Input: part model. Units: mm. Frame: model coordinates. A direction names the side the tool comes from. Round coordinates to 2 decimals unless told otherwise and drop trailing zeros. Order: outer loops, then holes, each group sorted by start corner. A loop starts at its lowest first (then second) coordinate and runs counter-clockwise, first axis right, second up. Notation, with made-up numbers: M 28.5,25.25 L 62.5,25.25 A25 cw 62.5,41.25 Z; hole C -14.75,-20.75 d11. An arc over 180 degrees is marked long. One line per question, with ' | ' between items.
```python
from build123d import *

# Parameters (mm, degrees)
SKETCH1_W           = 30
SKETCH1_H           = 15
SKETCH1_R           = 1.5
SKETCH1_W_2         = 15
SKETCH1_H_2         = 17
SKETCH1_R_2         = 5
BOSS_EXTRUDE1_DEPTH = 5
SKETCH3_R           = 5
BOSS_EXTRUDE2_DEPTH = 15


with BuildPart() as part:
    # Sketch1 → Boss-Extrude1 (new body)
    # profile 1 of 3: a face of its own
    with BuildSketch(Plane(origin=(0, 0, 0), x_dir=(1, 0, 0), z_dir=(0, 1, 0))):
        with Locations((-15, -7.5)):
            Rectangle(SKETCH1_W, SKETCH1_H)
        with Locations(Location((-5, -7.5, 0), (0, 0, 270))):
            Circle(SKETCH1_R, mode=Mode.SUBTRACT)
        with Locations(Location((-25, -7.5, 0), (0, 0, 270))):
            Circle(SKETCH1_R, mode=Mode.SUBTRACT)
    # profile 2 of 3: a face of its own
    with BuildSketch(Plane(origin=(0, 0, 0), x_dir=(1, 0, 0), z_dir=(0, 1, 0))):
        with Locations((-15, 8.5)):
            Rectangle(SKETCH1_W_2, SKETCH1_H_2)
        with Locations((-15, 9)):
            Circle(SKETCH1_R_2, mode=Mode.SUBTRACT)
    # profile 3 of 3: a face of its own
    with BuildSketch(Plane(origin=(0, 0, 0), x_dir=(1, 0, 0), z_dir=(0, 1, 0))):
        with Locations((-15, 9)):
            Circle(SKETCH1_R_2)
    extrude(amount=BOSS_EXTRUDE1_DEPTH)

    # Sketch3 → Boss-Extrude2 (add)
    with BuildSketch(Plane.XZ):
        with Locations(Location((-15, -9, 0), (0, 0, 270))):
            Circle(SKETCH3_R)
    extrude(amount=BOSS_EXTRUDE2_DEPTH)


solid = part.part
```
Item 1: Line query: line 1 along X through (y, z) = (3.4, 7.5); line 2 along Y through (x, z) = (-26, 3.5); line 3 along X through (y, z) = (1.5, -1.5). Output: solid intervals per line, ascending. Write a range as from..to.
Report:
line 1: -30..-26.5, -23.5..-6.5, -3.5..0 | line 2: 0..5 | line 3: -22.5..-7.5
Item 2: Mould query, pull axis Z, two halves, no side actions, for faces 1 (the cylindrical face through (-5, 2, 6)), 2 (the flat face through (-4, 2, 0)), 3 (the flat face through (-15, -15, -9)), 4 (the cylindrical face through (-23.513, 2.465, 7.305)). Classes: +Z half, -Z half, draft (parallel to the pull), parting line (faces both ways), or undercut.
Report:
face 1: undercut | face 2: -Z half | face 3: draft | face 4: undercut
Item 3: Section query B-B, the plane z = -9. Return loops of the section in (x, y).
Report:
outline: M -22.5,0 L -20,0 L -20,-15 L -10,-15 L -10,0 L -7.5,0 L -7.5,5 L -22.5,5 Z
Item 4: Section query C-C, the plane z = 7.5. Return loops of the section in (x, y).
Report:
outline: M -30,0 L -26.5,0 L -26.5,5 L -30,5 Z; M -23.5,0 L -6.5,0 L -6.5,5 L -23.5,5 Z; M -3.5,0 L 0,0 L 0,5 L -3.5,5 Z
Item 5: First-contact query: pin 1 (3.5 mm diameter, centred on x = -25, z = 7.5, fed in from -Y); pin 2 (1.5 mm diameter, centred on x = -27.5, y = 2, fed in from -Z); pin 3 (2.5 mm diameter, centred on y = 2, z = -6.5, fed in from +X). Flat tips, straight axial feed; report the tip coordinate or a pass-through.
Report:
pin 1: y = 0 | pin 2: z = 0 | pin 3: x = -7.5
Item 6: Section query A-A, the plane x = -5. Return loops of the section in (y, z), plus the area to 3 significant figures.
Report:
outline: M 0,0 L 5,0 L 5,6 L 0,6 Z; M 0,9 L 5,9 L 5,15 L 0,15 Z | area: 60.0 mm²
Item 7: Section query D-D, the plane y = -7. Return loops of the section in (x, z), plus the area to 3 significant figures.
Report:
outline: C -15,-9 d10 | area: 78.5 mm²
Item 8: Access query for faces 5 (the flat face through (-15, 2, -17)), 6 (the flat face through (-26, 2, 0)), 7 (the cylindrical face through (-19.436, -7.395, -11.307)), 8 (the flat face through (-7.5, 2, -8)), 9 (the flat face through (-15, 2, 15)). Directions: +Z, -Z, +X, -X, +Y, -Y. A direction counts if a zero-diameter tool reaches every point of the face in a straight line with its end or side. Return the directions, or none.
Report:
face 5: -Z, +X, -X, +Y, -Y | face 6: -Z, -X, +Y, -Y | face 7: -Y | face 8: -Z, +X, +Y, -Y | face 9: +Z, +X, -X, +Y, -Y
